from build123d import *

# Parameters (mm, degrees)
SKETCH_W   = 60
SKETCH_H   = 50
SKETCH_R   = 2.5
SKETCH_R_2 = 16
PAD_DEPTH  = 20
FILLET_R   = 5


with BuildPart() as part:
    # Sketch → Pad (new body)
    with BuildSketch(Plane.XY):
        Rectangle(SKETCH_W, SKETCH_H)
        with Locations((0, 20)):
            Circle(SKETCH_R, mode=Mode.SUBTRACT)
        with Locations((-20, 10)):
            Circle(SKETCH_R, mode=Mode.SUBTRACT)
        with Locations((-20, -10)):
            Circle(SKETCH_R, mode=Mode.SUBTRACT)
        with Locations((20, -10)):
            Circle(SKETCH_R, mode=Mode.SUBTRACT)
        with Locations((20, 10)):
            Circle(SKETCH_R, mode=Mode.SUBTRACT)
        with Locations((0, -20)):
            Circle(SKETCH_R, mode=Mode.SUBTRACT)
        Circle(SKETCH_R_2, mode=Mode.SUBTRACT)
    extrude(amount=PAD_DEPTH)

    # Fillet
    fillet_edges = [part.edges().sort_by_distance(p)[0] for p in [
        (30, 25, 10),
        (30, -25, 10),
        (-30, -25, 10),
        (-30, 25, 10),
    ]]
    fillet(fillet_edges, radius=FILLET_R)


solid = part.part
Geometry: final body of the model. Coordinates: model frame, mm. Round coordinates to 2 decimals unless told otherwise and drop trailing zeros. Order: outer loops, then holes, each group sorted by start corner. A loop starts at its lowest first (then second) coordinate and runs counter-clockwise, first axis right, second up.
Q1. Mould query, pull axis X, two halves, no side actions, for faces 1 (the face through (18, 8.5, 9.9)), 2 (the face through (0, 25, 10)), 3 (the face through (-29, -23, 10)). Classes: released by +X, released by -X, zero draft, split by the parting line, or undercut.
Result sheet:
face 1: undercut
face 2: zero draft
face 3: released by -X
Q2. Section C-C, the plane z = 13. Output: boundary loops of the cut face in (x, y).
Result sheet:
outline: (-30, -20) arc R5 ccw to (-25, -25) - (25, -25) arc R5 ccw to (30, -20) - (30, 20) arc R5 ccw to (25, 25) - (-25, 25) arc R5 ccw to (-30, 20) - close; hole circle Ø5 at (-20, -10); hole circle Ø5 at (-20, 10); hole circle Ø32 at (0, 0); hole circle Ø5 at (0, -20); hole circle Ø5 at (0, 20); hole circle Ø5 at (20, -10); hole circle Ø5 at (20, 10)
Q3. Section A-A, the plane y = 18.5. Output: boundary loops of the cut face in (x, z).
Result sheet:
outline: (-30, 0) - (-2, 0) - (-2, 20) - (-30, 20) - close; (2, 0) - (30, 0) - (30, 20) - (2, 20) - close
Q4. Section B-B, the plane x = 20. Output: boundary loops of the cut face in (y, z).
Result sheet:
outline: (-25, 0) - (-12.5, 0) - (-12.5, 20) - (-25, 20) - close; (-7.5, 0) - (7.5, 0) - (7.5, 20) - (-7.5, 20) - close; (12.5, 0) - (25, 0) - (25, 20) - (12.5, 20) - close
Q5. Section D-D, the plane x = 0. Output: boundary loops of the cut face in (y, z), and give its area (3 significant figures).
Result sheet:
outline: (-25, 0) - (-22.5, 0) - (-22.5, 20) - (-25, 20) - close; (-17.5, 0) - (-16, 0) - (-16, 20) - (-17.5, 20) - close; (16, 0) - (17.5, 0) - (17.5, 20) - (16, 20) - close; (22.5, 0) - (25, 0) - (25, 20) - (22.5, 20) - close
area: 160 mm2
Q6. Material intervals for probe 1 along Y at (x, z) = (-20, 5); probe 2 along Y at (x, z) = (0, 8.25); probe 3 along X at (y, z) = (-8.5, 11.25), sorted ascending.
Result sheet:
probe 1: y = -25 to -12.5, -7.5 to 7.5, 12.5 to 25
probe 2: y = -25 to -22.5, -17.5 to -16, 16 to 17.5, 22.5 to 25
probe 3: x = -30 to -22, -18 to -13.56, 13.56 to 18, 22 to 30
